from build123d import *

# Parameters (mm, degrees)
SKETCH1_R           = 9.5
SKETCH1_R_2         = 6.35
BOSS_EXTRUDE1_DEPTH = 26.5
SKETCH2_W           = 38
SKETCH2_H           = 12.5
CUT_EXTRUDE1_DEPTH  = 106.917446478
CUT_EXTRUDE3_START  = -6
CUT_EXTRUDE3_DEPTH  = 6
SKETCH6_R           = 6.35
CUT_EXTRUDE4_DEPTH  = 6
CUT_EXTRUDE6_DEPTH  = 5
CUT_EXTRUDE6_DRAFT  = -5
CUT_EXTRUDE7_DEPTH  = 5
CUT_EXTRUDE7_DRAFT  = -5


with BuildPart() as part:
    # Sketch1 → Boss-Extrude1 (new body)
    with BuildSketch(Plane.XY):
        with BuildLine():
            ThreePointArc((-19.80444005, 17.20999027), (-13.118685251, 4.903639601), (0, 0))
            Line((0, 0), (62, 0))
            Line((62, 0), (62, 13.5))
            Line((62, 13.5), (40, 13.5))
            ThreePointArc((40, 13.5), (33.5, 20), (40, 26.5))
            Line((40, 26.5), (62, 26.5))
            Line((62, 26.5), (62, 36.026416032))
            ThreePointArc((62, 36.026416032), (25.339969654, 45.733644305), (-0.177612992, 73.787896774))
            ThreePointArc((-0.177612992, 73.787896774), (-16.854632867, 81.076848535), (-26.639963888, 65.730868394))
            Line((-26.639963888, 65.730868394), (-19.80444005, 17.20999027))
        make_face()
        with Locations((0, 20)):
            Circle(SKETCH1_R, mode=Mode.SUBTRACT)
        with Locations((-12.776855853, 67.683875204)):
            Circle(SKETCH1_R_2, mode=Mode.SUBTRACT)
    extrude(amount=BOSS_EXTRUDE1_DEPTH)

    # Sketch2 → Cut-Extrude1 (cut, through all)
    with BuildSketch(Plane(origin=(0, 0, 0), x_dir=(1, 0, 0), z_dir=(0, 1, 0))):
        with Locations((43, -13.25)):
            Rectangle(SKETCH2_W, SKETCH2_H)
    extrude(amount=CUT_EXTRUDE1_DEPTH, mode=Mode.SUBTRACT)

    # Sketch3 → Cut-Extrude3 (cut)
    with BuildSketch(Plane.XY.offset(26.5).offset(CUT_EXTRUDE3_START)):
        with BuildLine():
            Line((3.956344678, 58.683875204), (9.868578653, 58.683875204))
            ThreePointArc((9.868578653, 58.683875204), (4.331951234, 65.89431889), (-0.177612992, 73.787896774))
            ThreePointArc((-0.177612992, 73.787896774), (-16.854632867, 81.076848535), (-26.639963888, 65.730868394))
            Line((-26.639963888, 65.730868394), (-24.848047694, 53.011236467))
            ThreePointArc((-24.848047694, 53.011236467), (-9.105576946, 49.041940992), (3.956344678, 58.683875204))
        make_face()
    extrude(amount=CUT_EXTRUDE3_DEPTH, mode=Mode.SUBTRACT)

    # Sketch6 → Cut-Extrude4 (cut)
    with BuildSketch(Plane(origin=(0, 0, 0), x_dir=(-1, 0, 0), z_dir=(0, 0, -1))):
        with BuildLine():
            Line((-9.868578653, 58.683875204), (-3.956344678, 58.683875204))
            ThreePointArc((-3.956344678, 58.683875204), (9.105576946, 49.041940992), (24.848047694, 53.011236467))
            Line((24.848047694, 53.011236467), (26.639963888, 65.730868394))
            ThreePointArc((26.639963888, 65.730868394), (16.854632867, 81.076848535), (0.177612992, 73.787896774))
            ThreePointArc((0.177612992, 73.787896774), (-4.331951234, 65.89431889), (-9.868578653, 58.683875204))
        make_face()
        with Locations((12.776855853, 67.683875204)):
            Circle(SKETCH6_R, mode=Mode.SUBTRACT)
    extrude(amount=-CUT_EXTRUDE4_DEPTH, mode=Mode.SUBTRACT)


with BuildPart() as cut_extrude6_tool:
    # Sketch7 → Cut-Extrude6 (with draft: the straight prism first)
    with BuildSketch(Plane.XY.offset(26.5)):
        with BuildLine():
            Line((8.973709214, 56.683875204), (5.111687967, 56.683875204))
            ThreePointArc((5.111687967, 56.683875204), (-7.062338313, 47.476344695), (-22.255412032, 48.944692384))
            Line((-22.255412032, 48.944692384), (-17.823996045, 17.488991243))
            ThreePointArc((-17.823996045, 17.488991243), (-11.806816725, 6.413275641), (0, 2))
            Line((0, 2), (60, 2))
            Line((60, 2), (60, 11.5))
            Line((60, 11.5), (40, 11.5))
            ThreePointArc((40, 11.5), (31.5, 20), (40, 28.5))
            Line((40, 28.5), (60, 28.5))
            Line((60, 28.5), (60, 34.000102209))
            ThreePointArc((60, 34.000102209), (32.089615412, 39.94948966), (8.973709214, 56.683875204))
        make_face()
    extrude(amount=-CUT_EXTRUDE6_DEPTH)
    # Cut-Extrude6: the draft: its side faces are tilted about the plane it starts from
    cut_extrude6_sides = [cut_extrude6_tool.faces().sort_by_distance(p)[0] for p in [
        (7.042698591, 56.683875204, 24),
        (-7.062338313, 47.476344695, 24),
        (-20.039704038, 33.216841814, 24),
        (-11.806816725, 6.413275641, 24),
        (30, 2, 24),
        (60, 6.75, 24),
        (50, 11.5, 24),
        (31.5, 20, 24),
        (50, 28.5, 24),
        (60, 31.250051104, 24),
        (32.089615412, 39.94948966, 24),
    ]]
    draft(cut_extrude6_sides, Plane.XY.offset(26.5), CUT_EXTRUDE6_DRAFT)


with BuildPart() as part_1:
    add(part.part)

    # Cut-Extrude6: cut by cut_extrude6_tool
    add(cut_extrude6_tool.part, mode=Mode.SUBTRACT)


with BuildPart() as cut_extrude7_tool:
    # Sketch8 → Cut-Extrude7 (with draft: the straight prism first)
    with BuildSketch(Plane(origin=(0, 0, 0), x_dir=(-1, 0, 0), z_dir=(0, 0, -1))):
        with BuildLine():
            Line((-5.111687967, 56.683875204), (-8.973709214, 56.683875204))
            ThreePointArc((-8.973709214, 56.683875204), (-32.089615412, 39.94948966), (-60, 34.000102209))
            Line((-60, 34.000102209), (-60, 28.5))
            Line((-60, 28.5), (-40, 28.5))
            ThreePointArc((-40, 28.5), (-31.5, 20), (-40, 11.5))
            Line((-40, 11.5), (-60, 11.5))
            Line((-60, 11.5), (-60, 2))
            Line((-60, 2), (0, 2))
            ThreePointArc((0, 2), (11.806816725, 6.413275641), (17.823996045, 17.488991243))
            Line((17.823996045, 17.488991243), (22.255412032, 48.944692384))
            ThreePointArc((22.255412032, 48.944692384), (7.062338313, 47.476344695), (-5.111687967, 56.683875204))
        make_face()
    extrude(amount=-CUT_EXTRUDE7_DEPTH)
    # Cut-Extrude7: the draft: its side faces are tilted about the plane it starts from
    cut_extrude7_sides = [cut_extrude7_tool.faces().sort_by_distance(p)[0] for p in [
        (7.042698591, 56.683875204, 2.5),
        (32.089615412, 39.94948966, 2.5),
        (60, 31.250051104, 2.5),
        (50, 28.5, 2.5),
        (31.5, 20, 2.5),
        (50, 11.5, 2.5),
        (60, 6.75, 2.5),
        (30, 2, 2.5),
        (-11.806816725, 6.413275641, 2.5),
        (-20.039704038, 33.216841814, 2.5),
        (-7.062338313, 47.476344695, 2.5),
    ]]
    draft(cut_extrude7_sides, Plane(origin=(0, 0, 0), x_dir=(-1, 0, 0), z_dir=(0, 0, -1)), CUT_EXTRUDE7_DRAFT)


with BuildPart() as part_2:
    add(part_1.part)

    # Cut-Extrude7: cut by cut_extrude7_tool
    add(cut_extrude7_tool.part, mode=Mode.SUBTRACT)


solid = part_2.part
Could you check a few things on this model? Use its own coordinates, in mm. A direction names the side the tool comes from. Give positions to 0.01 mm unless a question says otherwise; leave off trailing zeros. Loops run counter-clockwise (first coordinate to the right, second up) from the corner with the lowest first, then second, coordinate; pieces in that order, holes last. Notation, with made-up numbers: (12.5, 53.25) -> (51.5, 53.25) arc R17 cw to (51.5, 76.25) -> close; hole circle Ø8 at (85.25, 1.5). An arc over 180 degrees is marked (long way). Return JSON: item names as keys, results as strings.
Item 1: If we section it at A-A on z = 2: List the corners of the cut face in (x, y) for me, plus the area to 3 significant figures.
Geometry results:
{"outline": "(-24.85, 53.01) -> (-19.8, 17.21) arc R20 ccw to (0, 0) -> (62, 0) -> (62, 13.5) -> (40, 13.5) arc R6.5 cw to (40, 26.5) -> (62, 26.5) -> (62, 36.03) arc R67 cw to (9.87, 58.68) -> (3.96, 58.68) arc R19 cw to start; hole (-22.04, 48.64) -> (-17.65, 17.51) arc R17.83 ccw to (0, 2.17) -> (59.83, 2.17) -> (59.83, 11.33) -> (40, 11.33) arc R8.67 cw to (40, 28.67) -> (59.83, 28.67) -> (59.83, 33.83) arc R69.17 cw to (8.9, 56.51) -> (5.21, 56.51) arc R21.17 cw to start", "area": "655 mm²"}
Item 2: I'm going to push flat-ended pins straight in: pin 1 (7.5 mm diameter, centred on x = -12.78, y = 67.68, fed in from +Z); pin 2 (5.5 mm diameter, centred on x = 50.5, z = 2.5, fed in from +Y); pin 3 (10 mm diameter, centred on x = -0.5, y = 67.5, fed in from -Z); pin 4 (2 mm diameter, centred on x = 49, z = 24, fed in from +Y). Where does each tip first touch, or does it pass through?
Geometry results:
{"pin 1": "passes through", "pin 2": "stops at y = 37.15", "pin 3": "stops at z = 6", "pin 4": "stops at y = 37.11"}
Item 3: If we section it at C-C on y = 20: List the corners of the cut face in (x, z) for me.
Geometry results:
{"outline": "(-20.2, 0) -> (-18.18, 0) -> (-17.74, 5) -> (-9.5, 5) -> (-9.5, 21.5) -> (-17.74, 21.5) -> (-18.18, 26.5) -> (-20.2, 26.5) -> close; (9.5, 5) -> (31.06, 5) -> (31.5, 0) -> (33.5, 0) -> (33.5, 7) -> (24, 7) -> (24, 19.5) -> (33.5, 19.5) -> (33.5, 26.5) -> (31.5, 26.5) -> (31.06, 21.5) -> (9.5, 21.5) -> close"}
Item 4: I need wall thicknesses on L1, parallel to Z at x = -20.5, y = 73.5; L2, parallel to Z at x = -14, y = 17; L3, parallel to X at y = 63, z = 17. Which ranges of each line are inside material? Lowest first, please. Write a range as from..to.
Geometry results:
{"L1": "z = 6..20.5", "L2": "z = 5..21.5", "L3": "x = -26.26..-17.06, -8.49..6.37"}
Item 5: If we section it at D-D on x = 43.5: Count the separate pieces of the cut face and the enclosed holes in it, plus the area to 3 significant figures.
Geometry results:
{"separate pieces": "4", "enclosed holes": "0", "area": "190 mm²"}
Item 6: If we section it at B-B on z = 15: List the corners of the cut face in (x, y) for me.
Geometry results:
{"outline": "(-26.64, 65.73) -> (-19.8, 17.21) arc R20 ccw to (0, 0) -> (24, 0) -> (24, 46.57) arc R67 cw to (-0.18, 73.79) arc R14 ccw to start; hole circle Ø12.7 at (-12.78, 67.68); hole circle Ø19 at (0, 20)"}
Item 7: Which directions (+Z, -Z, +X, -X, +Y, -Y) give clear straight access to the entire face, cutting with the end or side of a thin tool? Please do faces 5 (the conical face through (-11.53, 6.46, 2.47)), 6 (the flat face through (51, 26.5, 23)), 7 (the flat face through (7, 58.684, 3)), 8 (the conical face through (31.286, 19.808, 24.035)), 9 (the flat face through (24, 23, 13)).
Geometry results:
{"face 5": "-Z", "face 6": "+Z, -Z, +X", "face 7": "-Z, +X, -X, +Y", "face 8": "+Z", "face 9": "+X, +Y, -Y"}
Item 8: We'd pull the mould along Y, two halves only. Please class faces 1 (the conical face through (32.37, 39.59, 24.04)), 2 (the flat face through (23.7, 0, 13.1)), 3 (the flat face through (-9, 62, 20.5)), 4 (the cylindrical face through (18.76, 50.29, 13.06)): +Y half, -Y half, draft (parallel to the pull), parting line (faces both ways), or undercut.
Geometry results:
{"face 1": "undercut", "face 2": "-Y half", "face 3": "draft", "face 4": "+Y half"}
